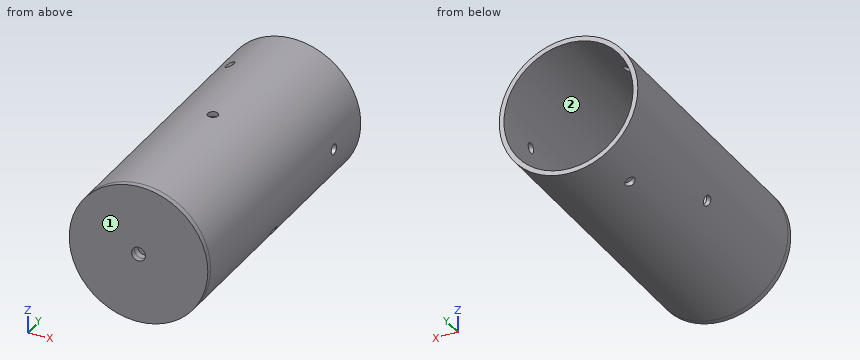
Autodesk Inventor part; units mm, degrees
ref_plane "Work Plane1" through (0, 95.06, 0) normal (0, 1, 0) x (1, 0, 0)
ref_plane "Work Plane2" through (0, 55.16, 0) normal (0, 1, 0) x (1, 0, 0)
ref_plane "YZ Plane" through (0, 0, 0) normal (1, 0, 0) x (0, 1, 0)
sketch "Sketch1" plane through (0, 0, 0) normal (0, 1, 0) x (-1, 0, 0)
  circle A0 centre (0, 0) radius 27.31
  circle A1 centre (0, 0) radius 25.445
  dimension "d0" = 54.62
  dimension "d1" = 50.89
extrude "Extrusion1" add sketch "Sketch1" along normal blind 115.81
sketch "Sketch2" plane through (0, 0, 0) normal (0, -1, 0) x (1, 0, 0)
  circle A0 centre (0, 0) radius 27.31
extrude "Extrusion2" add sketch "Sketch2" along normal blind 2.18
sketch "Sketch3" plane through (0, -2.18, 0) normal (0, -1, 0) x (1, 0, 0)
  circle A0 centre (0, 0) radius 2.75
  dimension "d6" = 5.5
extrude "Extrusion3" cut sketch "Sketch3" against normal up to surface (2.18 mm away)
sketch "Sketch4" plane through (0, 0, 0) normal (0, 1, 0) x (1, 0, 0)
  circle A0 centre (0, 0) radius 2.75
  circle A1 centre (0, 0) radius 25.445
  circle A2 centre (0, 0) radius 2.75
extrude "Extrusion4" add sketch "Sketch4" along normal blind 2.56
ref_plane "Work Plane1" through (0, 95.06, 0) normal (0, 1, 0) x (1, 0, 0)
sketch "Sketch6" plane through (0, 95.06, 0) normal (0, 1, 0) x (1, 0, 0)
  circle A0 centre (0, 0) radius 27.31
  point P0 (27.31, 0)
  point P1 (-13.655, 23.6512)
  point P2 (-13.655, -23.6512)
  dimension "d18" = 360
hole "Hole1" at (-13.655, 95.06, -23.6512) direction (0.5, 0, 0.866) diameter 4.1 depth 2
hole "Hole2" at (-13.655, 95.06, 23.6512) direction (0.5, 0, -0.866) diameter 4.1 depth 2
hole "Hole3" at (27.31, 95.06, 0) direction (-1, 0, 0) diameter 4.1 depth 2
ref_plane "Work Plane2" through (0, 55.16, 0) normal (0, 1, 0) x (1, 0, 0)
sketch "Sketch7" plane through (0, 55.16, 0) normal (0, 1, 0) x (1, 0, 0)
  circle A0 centre (0, 0) radius 27.31
  point P0 (0, -27.31)
  point P1 (23.6512, 13.655)
  point P2 (-23.6512, 13.655)
  dimension "d50" = 360
hole "Hole4" at (23.6512, 55.16, -13.655) direction (-0.866, 0, 0.5) diameter 4.1 depth 2
hole "Hole5" at (0, 55.16, 27.31) direction (0, 0, -1) diameter 4.1 depth 2
hole "Hole6" at (-23.6512, 55.16, -13.655) direction (0.866, 0, 0.5) diameter 4.1 depth 2
sketch "Sketch8" plane through (0, 2.56, 0) normal (0, 1, 0) x (1, 0, 0)
  circle A0 centre (0, 0) radius 2.75
  circle A1 centre (0, 0) radius 2.75
  line L0 (-4.8047, 0) -> (-2.4023, 4.161)
  line L1 (-2.4023, 4.161) -> (2.4023, 4.161)
  line L2 (2.4023, 4.161) -> (4.8047, 0)
  line L3 (4.8047, 0) -> (2.4023, -4.161)
  line L4 (2.4023, -4.161) -> (-2.4023, -4.161)
  line L5 (-2.4023, -4.161) -> (-4.8047, 0)
extrude "Extrusion5" add sketch "Sketch8" along normal blind 22.06 contours A0
extrude "Extrusion6" add sketch "Sketch8" along normal blind 3.175
ref_plane "Work Plane3" through (-2.4023, 2.56, -0.919) normal (0, 0, 1) x (1, 0, 0)
properties part number "avbay"
The model under review builds one solid part; all positions refer to its coordinate system, in mm. Face numbers are marked on the shaded views. Give positions to 0.01 mm unless a question says otherwise; leave off trailing zeros. Write each loop counter-clockwise with the first axis right and the second up, starting at its lowest first coordinate (ties: lowest second). Pieces come first, ordered by that corner, then holes. Notation, with made-up numbers: M 80,0 L 124,0 A13 cw 124,5 Z; hole C 82.25,37 d9. An arc over 180 degrees is marked long. Answer in a Markdown table with one row per item.
Item 1: Add section C-C on y = 40. Give the boundary of the cut face in (x, z) (3 decimals).
Check sheet entries:
| item | result |
|---|---|
| outline | C 0,0 d54.62; hole C 0,0 d50.89 |
Item 2: For line 1 along X through (y, z) = (32.5, 1); line 2 along Z through (x, y) = (0, 0); line 3 along Z through (x, y) = (0, 53) (3 decimals), list the stretches that pass through material, from the lowest coordinate up.
Check sheet entries:
| item | result |
|---|---|
| line 1 | -27.29 to -25.43, 25.43 to 27.29 |
| line 2 | -27.31 to -2.75, 2.75 to 27.31 |
| line 3 | -27.31 to -25.445, 25.445 to 27.31 |
Item 3: For P1, Ø2.5, axis at x = 0, y = 55.16, coming from the -Z side; P2, Ø1, axis at x = 0.5, y = 4, coming from the +Z side; P3, Ø8, axis at y = 14.5, z = -12.5, coming from the -X side, all flat-tipped, find the tip position at first contact; note any pin that passes through.
Check sheet entries:
| item | result |
|---|---|
| P1 | z = -27.31 |
| P2 | z = 27.31 |
| P3 | x = -25.95 |
Item 4: Add section B-B on y = 55.16. Give the boundary of the cut face in (x, z) (3 decimals).
Check sheet entries:
| item | result |
|---|---|
| outline | M -24.609,-11.841 L -22.989,-10.906 A25.445 cw -2.05,25.362 L -2.05,27.233 A27.31 ccw Z; M -22.559,-15.392 A27.31 ccw 22.559,-15.392 L 20.939,-14.456 A25.445 cw -20.939,-14.456 Z; M 2.05,25.362 A25.445 cw 22.989,-10.906 L 24.609,-11.841 A27.31 ccw 2.05,27.233 Z |
Item 5: Draft analysis for pull direction X (two halves, no side actions). For the marked faces 1 and 2, state which applies: +X half, -X half, draft (parallel to the pull), parting line (faces both ways), or undercut.
Check sheet entries:
| item | result |
|---|---|
| face 1 | draft |
| face 2 | undercut |
Item 6: Add section A-A on x = 0. Give the boundary of the cut face in (y, z) (3 decimals), plus the area to 3 significant figures.
Check sheet entries:
| item | result |
|---|---|
| outline | M -2.18,-27.31 L 115.81,-27.31 L 115.81,-25.445 L 2.56,-25.445 L 2.56,-4.161 L 5.735,-4.161 L 5.735,-2.75 L 24.62,-2.75 L 24.62,2.75 L 5.735,2.75 L 5.735,4.161 L 2.56,4.161 L 2.56,25.445 L 53.11,25.445 L 53.11,27.31 L -2.18,27.31 L -2.18,2.75 L 2.56,2.75 L 2.56,-2.75 L -2.18,-2.75 Z; M 57.21,25.445 L 115.81,25.445 L 115.81,27.31 L 57.21,27.31 Z |
| area | 778 mm2 |
Item 7: Add section D-D on z = 10. Give the boundary of the cut face in (x, y), plus the area to 3 significant figures.
Check sheet entries:
| item | result |
|---|---|
| outline | M -25.41,-2.18 L 25.41,-2.18 L 25.41,115.81 L 23.4,115.81 L 23.4,2.56 L -23.4,2.56 L -23.4,115.81 L -25.41,115.81 Z |
| area | 697 mm2 |
